```python
from build123d import *

# Parameters (mm, degrees)
F1_DEPTH = 10
F3_DEPTH = 10.001
F4_W     = 8
F4_H     = 8
F4_H_2   = 8.779348
F5_DEPTH = 10.001


with BuildPart() as f1:
    # F0 (on Front) → F1 (new body)
    with BuildSketch(Plane.XZ):
        with BuildLine():
            ThreePointArc((-70.378245, 42.093974), (-67.611515, 36.816708), (-68.337629, 30.902564))
            ThreePointArc((-68.337629, 30.902564), (0, -75), (68.337629, 30.902564))
            ThreePointArc((68.337629, 30.902564), (67.611515, 36.816708), (70.378245, 42.093974))
            Line((70.378245, 42.093974), (70.710678, 42.426407))
            ThreePointArc((70.710678, 42.426407), (73.63961, 49.497475), (70.710678, 56.568542))
            Line((70.710678, 56.568542), (56.568542, 70.710678))
            ThreePointArc((56.568542, 70.710678), (49.497475, 73.63961), (42.426407, 70.710678))
            Line((42.426407, 70.710678), (42.093974, 70.378245))
            ThreePointArc((42.093974, 70.378245), (36.816708, 67.611515), (30.902564, 68.337629))
            ThreePointArc((30.902564, 68.337629), (0, 75), (-30.902564, 68.337629))
            ThreePointArc((-30.902564, 68.337629), (-36.816708, 67.611515), (-42.093974, 70.378245))
            Line((-42.093974, 70.378245), (-42.426407, 70.710678))
            ThreePointArc((-42.426407, 70.710678), (-49.497475, 73.63961), (-56.568542, 70.710678))
            Line((-56.568542, 70.710678), (-70.710678, 56.568542))
            ThreePointArc((-70.710678, 56.568542), (-73.63961, 49.497475), (-70.710678, 42.426407))
            Line((-70.710678, 42.426407), (-70.378245, 42.093974))
        make_face()
    extrude(amount=F1_DEPTH)

    # F2 (on face) → F3 (cut, through all)
    with BuildSketch(Plane(origin=(0, 0, 0), x_dir=(-1, 0, 0), z_dir=(0, 1, 0))):
        with BuildLine():
            ThreePointArc((-50.911688, 42.426407), (-42.426407, 42.426407), (-42.426407, 50.911688))
            Line((-42.426407, 50.911688), (-48.083261, 56.568542))
            ThreePointArc((-48.083261, 56.568542), (-56.568542, 56.568542), (-56.568542, 48.083261))
            Line((-56.568542, 48.083261), (-50.911688, 42.426407))
        make_face()
        with BuildLine():
            Line((50.911688, 42.426407), (56.568542, 48.083261))
            ThreePointArc((56.568542, 48.083261), (56.568542, 56.568542), (48.083261, 56.568542))
            Line((48.083261, 56.568542), (42.426407, 50.911688))
            ThreePointArc((42.426407, 50.911688), (42.426407, 42.426407), (50.911688, 42.426407))
        make_face()
    extrude(amount=-F3_DEPTH, mode=Mode.SUBTRACT)

    # F4 (on face) → F5 (cut, through all)
    with BuildSketch(Plane.XZ.offset(10)):
        with Locations((64, 0)):
            Rectangle(F4_W, F4_H)
        with Locations((0, 64)):
            Rectangle(F4_W, F4_H)
        with Locations((0, -64)):
            Rectangle(F4_W, F4_H)
        with Locations((-64, 0)):
            Rectangle(F4_W, F4_H)
        with Locations((45.254834, -45.254834)):
            Rectangle(F4_W, F4_H_2)
        with Locations((-45.254834, -45.254834)):
            Rectangle(F4_W, F4_H_2)
    extrude(amount=-F5_DEPTH, mode=Mode.SUBTRACT)


solid = f1.part
```
Can you work these out from the model? Positions are in its coordinate system, mm. A direction names the side the tool comes from. Coordinates: 2 decimals unless noted, no trailing zeros. Loops run counter-clockwise (first coordinate to the right, second up) from the corner with the lowest first, then second, coordinate; pieces in that order, holes last. Notation, with made-up numbers: M 13,46.5 L 37,46.5 A17 cw 37,64.5 Z; hole C 88.5,8 d2. An arc over 180 degrees is marked long. Put each result on its own line as item: value. Start each with the question number.
(1) Will these pins go through, and if not, where does the flat tip stop? pin 1 Ø4 at (y, z) = (-3.5, 0) entering from +X; pin 2 Ø4 at (x, y) = (-62.5, -4.5) entering from +Z; pin 3 Ø1.5 at (y, z) = (-3.5, 48) entering from +X.
(2) Which directions (+Z, -Z, +X, -X, +Y, -Y) give clear straight access to the entire face, cutting with the end or side of a thin tool? Please do faces 1 (the face through (-63.54, -4.93, 63.74)), 2 (the face through (4, -5, -64)).
(3) Imagine slicing it at B-B on x = 0. List the corners of the cut face in (y, z) for me, and give its area (3 significant figures).
(4) Imagine slicing it at A-A on z = 0. List the corners of the cut face in (x, y) for me, and give its area (3 significant figures).
(5) I need wall thicknesses on probe 1 along X at (y, z) = (-3.75, 2); probe 2 along Z at (x, y) = (-48, -3); probe 3 along X at (y, z) = (-3.25, 48). Which ranges of each line are inside material? Lowest first, please.
(6) Imagine slicing it at D-D on y = -6.5. Give the number of separate pieces and of enclosed holes in the cut face, and give its area (3 significant figures).
(7) Imagine slicing it at C-C on x = 54. List the corners of the cut face in (y, z) for me.
(8) We'd pull the mould along Z, two halves only. Please class faces 3 (the face through (63.74, -4.93, 63.54)), 4 (the face through (41.255, -5, -45)), 5 (the face through (45, -5, -49.645)): +Z half, -Z half, draft (parallel to the pull), parting line (faces both ways), or undercut.
Worked answers:
1. pin 1: stops at x = 75
1. pin 2: stops at z = 66.78
1. pin 3: stops at x = 73.61
2. face 1: +Z, -X, +Y, -Y
2. face 2: +Y, -Y
3. outline: M -10,-75 L 0,-75 L 0,-68 L -10,-68 Z; M -10,-60 L 0,-60 L 0,60 L -10,60 Z; M -10,68 L 0,68 L 0,75 L -10,75 Z
3. area: 1,340 mm2
4. outline: M -75,-10 L -68,-10 L -68,0 L -75,0 Z; M -60,-10 L 60,-10 L 60,0 L -60,0 Z; M 68,-10 L 75,-10 L 75,0 L 68,0 Z
4. area: 1,340 mm2
5. probe 1: x = -74.97 to -68, -60 to 60, 68 to 74.97
5. probe 2: z = -57.63 to -49.64, -40.87 to 40.82, 56.49 to 73.53
5. probe 3: x = -73.53 to -56.49, -40.82 to 40.82, 56.49 to 73.53
6. separate pieces: 1
6. enclosed holes: 8
6. area: 18,100 mm2
7. outline: M -10,-52.05 L 0,-52.05 L 0,45.51 L -10,45.51 Z; M -10,58.09 L 0,58.09 L 0,72.57 L -10,72.57 Z
8. face 3: +Z half
8. face 4: undercut
8. face 5: undercut
